```python
from build123d import *

# Parameters (mm, degrees)
EXTRUDE_1_DEPTH        = 25
SKETCH_2_W             = 4
SKETCH_2_H             = 4
EXTRUDE_2_DEPTH        = 30
PATTERN_LINEAR_1_COUNT = 5
PATTERN_LINEAR_1_PITCH = 5
FILLET_1_R             = 1


with BuildPart() as part:
    # 草图1 → 凸台-拉伸1 (new body)
    with BuildSketch(Plane.XY):
        Polygon((-10, 5), (-10, 12), (-3.333333333, 5), (-3.333333333, 12), (3.333333333, 5), (3.333333333, 12), (10, 5), (10, -5), (-10, -5), align=None)
    extrude(amount=EXTRUDE_1_DEPTH)

    # 草图2 → 凸台-拉伸2 (add)
    with BuildSketch(Plane.XZ.offset(5)):
        with Locations((-8, 23)):
            Rectangle(SKETCH_2_W, SKETCH_2_H)
    extrude_2 = extrude(amount=-EXTRUDE_2_DEPTH)

    # 阵列(线性)1: 凸台-拉伸2 ×5
    with Locations(*[(0, 0, -i * PATTERN_LINEAR_1_PITCH) for i in range(1, PATTERN_LINEAR_1_COUNT)]):
        add(extrude_2)

    # 圆角1
    fillet_1_edges = [part.edges().sort_by_distance(p)[0] for p in [
        (-10, 25, 3),
        (-8, 25, 5),
        (-6, 25, 3),
        (-8, 25, 1),
        (-10, 10, 25),
        (10, 0, 25),
        (-8, 25, 25),
        (-8, 25, 21),
        (-10, 25, 23),
        (-6, 25, 23),
        (-10, 25, 18),
        (-8, 25, 20),
        (-6, 25, 18),
        (-8, 25, 16),
        (-10, 25, 13),
        (-8, 25, 15),
        (-6, 25, 13),
        (-8, 25, 11),
        (10, 0, 0),
        (-10, 25, 8),
        (-8, 25, 10),
        (-6, 25, 8),
        (-8, 25, 6),
        (-10, 3.5, 0),
    ]]
    fillet(fillet_1_edges, radius=FILLET_1_R)


solid = part.part
```
CAD build for the part. Positions are in the model's coordinates, mm. A direction names the side the tool comes from. Round coordinates to 2 decimals unless told otherwise and drop trailing zeros. Order: outer loops, then holes, each group sorted by start corner. A loop starts at its lowest first (then second) coordinate and runs counter-clockwise, first axis right, second up.
Q1. Drop flat-ended pins along their axis: pin 1 (2 mm diameter, centred on y = 12, z = 8.5, fed in from +X); pin 2 (2 mm diameter, centred on x = -7.5, y = 19.5, fed in from -Z); pin 3 (1.2 mm diameter, centred on y = 19.5, z = 19, fed in from +X). Give the stop position or say it passes through.
Q2. Slice it at D-D (x = 2.75). Write the cut outline in (y, z), and give its area (3 significant figures).
Q3. Wall check: L1, parallel to X at y = 6.5, z = 5; L2, parallel to X at y = 5.75, z = 4.75; L3, parallel to X at y = 17.5, z = 3.75. Give the ranges that are in metal, low to high.
Q4. Which spindle directions (+Z, -Z, +X, -X, +Y, -Y) get a long thin tool onto all of the face, cutting with end or side? Do faces 1 (the flat face through (-6, 16, 3)), 2 (the cylindrical face through (-8, 24.6, 16.2)), 3 (the flat face through (-10, 10, 12)). Say none if no direction does.
Q5. Slice it at B-B (z = 18). Write the cut outline in (x, y), and give its area (3 significant figures).
Q6. Slice it at C-C (y = 9.75). State how many separate pieces and enclosed holes the cut face has, and give its area (3 significant figures).
Q7. Slice it at A-A (y = 16.5). Write the cut outline in (x, z), and give its area (3 significant figures).
Q8. Two-plate mould, pull along Z, no slides. Class faces 4 (the cylindrical face through (-7.479, 24.715, 24.699)), 5 (the cylindrical face through (-8, 24.6, 6.2)), 6 (the flat face through (-8, 25, 13)): pulls with the +Z half, pulls with the -Z half, needs draft (parallel to the pull), parting line crosses it, or undercut.
Results below:
1. pin 1: stops at x = 4.29
1. pin 2: stops at z = 1
1. pin 3: stops at x = -6
2. outline: (-5, 0) - (5.61, 0) - (5.61, 25) - (-5, 25) - close
2. area: 265 mm2
3. L1: x = -10 to -4.76, -3.33 to 1.9, 3.33 to 8.57
3. L2: x = -10 to -4.05, -3.33 to 2.62, 3.33 to 9.29
3. L3: x = -10 to -6
4. face 1: +Z, -Z, +Y
4. face 2: +X, -X, +Y
4. face 3: +Z, -Z, -X, +Y, -Y
5. outline: (-10, -5) - (10, -5) - (10, 5) - (3.33, 12) - (3.33, 5) - (-3.33, 12) - (-3.33, 5) - (-6, 7.8) - (-6, 24) arc R1 ccw to (-7, 25) - (-9, 25) arc R1 ccw to (-10, 24) - close
5. area: 330 mm2
6. separate pieces: 3
6. enclosed holes: 0
6. area: 197 mm2
7. outline: (-10, 1) - (-6, 1) - (-6, 5) - (-10, 5) - close; (-10, 6) - (-6, 6) - (-6, 10) - (-10, 10) - close; (-10, 11) - (-6, 11) - (-6, 15) - (-10, 15) - close; (-10, 16) - (-6, 16) - (-6, 20) - (-10, 20) - close; (-10, 21) - (-6, 21) - (-6, 25) - (-9, 25) arc R1 ccw to (-10, 24) - close
7. area: 79.8 mm2
8. face 4: pulls with the +Z half
8. face 5: undercut
8. face 6: needs draft
